```python
from build123d import *

# Parameters (mm, degrees)
SKETCH2_W                = 457.2
SKETCH2_H                = 609.6
SKETCH2_W_2              = 38.1
SKETCH2_H_2              = 38.1
SKETCH2_W_3              = 48.862926818
SKETCH2_H_3              = 48.862926818
BOSS_EXTRUDE1_DEPTH      = 17.78
SKETCH3_W                = 17.78
SKETCH3_H                = 609.6
BOSS_EXTRUDE2_DEPTH      = 381
BOSS_EXTRUDE3_DEPTH      = 17.78
BOSS_EXTRUDE3_DEPTH_BACK = 787.4
SKETCH4_W                = 38.1
SKETCH4_H                = 38.1
SKETCH4_W_2              = 48.862926818
SKETCH4_H_2              = 48.862926818


with BuildPart() as part:
    # Sketch2 → Boss-Extrude1 (new body)
    with BuildSketch(Plane(origin=(0, 0, 0), x_dir=(1, 0, 0), z_dir=(0, 1, 0))):
        Rectangle(SKETCH2_W, SKETCH2_H)
        with Locations((-158.75, 260.35)):
            Rectangle(SKETCH2_W_2, SKETCH2_H_2, mode=Mode.SUBTRACT)
        with Locations((-153.368536591, -254.968536591)):
            Rectangle(SKETCH2_W_3, SKETCH2_H_3, mode=Mode.SUBTRACT)
    extrude(amount=BOSS_EXTRUDE1_DEPTH)

    # Sketch3 → Boss-Extrude2 (add)
    with BuildSketch(Plane(origin=(0, 0, 0), x_dir=(1, 0, 0), z_dir=(0, 1, 0))):
        with Locations((219.71, 0)):
            Rectangle(SKETCH3_W, SKETCH3_H)
    extrude(amount=-BOSS_EXTRUDE2_DEPTH)

    # Sketch4 → Boss-Extrude3 (add, two sides: drawn at the far end of the back side and taken through both)
    with BuildSketch(Plane(origin=(0, 0, 0), x_dir=(1, 0, 0), z_dir=(0, 1, 0)).offset(-BOSS_EXTRUDE3_DEPTH_BACK)):
        with Locations((-158.75, 260.35)):
            Rectangle(SKETCH4_W, SKETCH4_H)
        with Locations((-153.368536591, -254.968536591)):
            Rectangle(SKETCH4_W_2, SKETCH4_H_2)
    extrude(amount=BOSS_EXTRUDE3_DEPTH + BOSS_EXTRUDE3_DEPTH_BACK)


solid = part.part
```
Can you work these out from the model? Positions are in its coordinate system, mm. A direction names the side the tool comes from. Coordinates: 2 decimals unless noted, no trailing zeros. Loops run counter-clockwise (first coordinate to the right, second up) from the corner with the lowest first, then second, coordinate; pieces in that order, holes last.
1) Imagine slicing it at A-A on y = -479.5. List the corners of the cut face in (x, z) for me.
2) I need wall thicknesses on probe 1 along X at (y, z) = (-331.5, 272.5); probe 2 along X at (y, z) = (-267.5, -266); probe 3 along Y at (x, z) = (24, 44). Which ranges of each line are inside material? Lowest first, please.
3) Imagine slicing it at B-B on y = -35.5. List the corners of the cut face in (x, z) for me.
4) Thinking about a two-plate mould opening in X: for faces 5 (the flat face through (-177.8, -399, 255)), 6 (the flat face through (-139.7, -399, -260)), 7 (the flat face through (-154, -399, 279.4)), which applies, pulls with the +X half, pulls with the -X half, needs draft (parallel to the pull), parting line crosses it, or undercut?
5) Imagine slicing it at D-D on z = -120.5. List the corners of the cut face in (x, y) for me, plus the area to 3 significant figures.
6) Which directions (+Z, -Z, +X, -X, +Y, -Y) give clear straight access to the entire face, cutting with the end or side of a thin tool? Please do faces 1 (the flat face through (-159, -399, -279.4)), 2 (the flat face through (210.82, -188, 4)), 3 (the flat face through (-154, -399, 230.537)), 4 (the flat face through (-177.8, -399, -260)).
7) For pin 1 (5 mm diameter, centred on x = -158, y = -129.5, fed in from -Z); pin 2 (10 mm diameter, centred on x = -150.5, y = -586, fed in from +Z); pin 3 (10 mm diameter, centred on y = -119.5, z = -34, fed in from -X), each with a flat end and sliding along its axis, tell me the tip position at first contact or that it passes through.
8) Imagine slicing it at C-C on x = -160.5. List the corners of the cut face in (y, z) for me, plus the area to 3 significant figures.
Completed:
1. outline: (-177.8, -279.4) - (-139.7, -279.4) - (-139.7, -241.3) - (-177.8, -241.3) - close; (-177.8, 230.54) - (-128.94, 230.54) - (-128.94, 279.4) - (-177.8, 279.4) - close
2. probe 1: x = -177.8 to -128.94, 210.82 to 228.6
2. probe 2: x = -177.8 to -139.7, 210.82 to 228.6
2. probe 3: y = 0 to 17.78
3. outline: (-177.8, -279.4) - (-139.7, -279.4) - (-139.7, -241.3) - (-177.8, -241.3) - close; (-177.8, 230.54) - (-128.94, 230.54) - (-128.94, 279.4) - (-177.8, 279.4) - close; (210.82, -304.8) - (228.6, -304.8) - (228.6, 304.8) - (210.82, 304.8) - close
4. face 5: pulls with the -X half
4. face 6: undercut
4. face 7: needs draft
5. outline: (-228.6, 0) - (210.82, 0) - (210.82, -381) - (228.6, -381) - (228.6, 17.78) - (-228.6, 17.78) - close
5. area: 14,900 mm2
6. face 1: -Z, -X, -Y
6. face 2: +Z, -Z, -Y
6. face 3: -X, -Y
6. face 4: +Z, -Z, -X, -Y
7. pin 1: stops at z = -279.4
7. pin 2: stops at z = 279.4
7. pin 3: stops at x = 210.82
8. outline: (-787.4, -279.4) - (0, -279.4) - (0, -304.8) - (17.78, -304.8) - (17.78, 304.8) - (0, 304.8) - (0, 279.4) - (-787.4, 279.4) - (-787.4, 230.54) - (0, 230.54) - (0, -241.3) - (-787.4, -241.3) - close
8. area: 79,300 mm2
